Build history of the part. All positions in model axes, mm. A direction names the side the tool comes from. Give positions to 0.01 mm unless a question says otherwise; leave off trailing zeros. Order: outer loops, then holes, each group sorted by start corner. A loop starts at its lowest first (then second) coordinate and runs counter-clockwise, first axis right, second up. Notation, with made-up numbers: (45, -9) - (61, -9) arc R22 ccw to (61, 28) - close; hole circle Ø10 at (74.5, 22.5). An arc over 180 degrees is marked (long way). Use a Markdown table: item, result. Add a question column.
(1) Mould opens along Z. For faces 1 (the face through (59.49, 0.14, -11.07)), 2 (the face through (54.933, 0.14, -0.52)), 3 (the face through (0, 10, 53)) say: +Z half, -Z half, draft (parallel to the pull), parting line (faces both ways), or undercut.
(2) Flat gauge pins, fed straight in: pin 1 (4.5 mm diameter, centred on x = 57.28, z = 0, fed in from +Y); pin 2 (4 mm diameter, centred on x = 53, y = 2, fed in from +Z); pin 3 (5.5 mm diameter, centred on x = -57.28, z = 0, fed in from -Y); pin 4 (19.5 mm diameter, centred on x = -37.5, z = -36.5, fed in from -Y). Where does each tip first touch, or does it go through?
(3) Wall check: line 1 (X direction, y = 2.5, z = 0); line 2 (Y direction, x = -51.5, z = 16); line 3 (Z direction, x = 35.5, y = -1.5). Give the ranges that are in metal, low to high.
(4) Slice it at B-B (x = -26.5). Write the cut outline in (y, z).
(5) Slice it at D-D (y = -1). Write the cut outline in (x, z), then the cut area to 3 significant figures.
(6) Slice it at C-C (z = -15). Write the cut outline in (x, y), then the cut area to 3 significant figures.
(7) Slice it at A-A (z = 0). Write the cut outline in (x, y), then the cut area to 3 significant figures.
(8) Which spindle directions (+Z, -Z, +X, -X, +Y, -Y) get a long thin tool onto all of the face, cutting with end or side? Do faces 4 (the face through (55, -2, -12.5)), 5 (the face through (-55, -2, -12.5)), 6 (the face through (-55, -2, 12.5)), 7 (the face through (15, 3, -52)), 8 (the face through (55, -2, 12.5)). Say none if no direction does.
from build123d import *

# Parameters (mm, degrees)
BOSS_EXTRUDE1_DEPTH      = 10
BOSS_EXTRUDE1_DEPTH_BACK = 5
SKETCH1_R                = 55
SKETCH1_R_2              = 52.5
CUT_EXTRUDE2_DEPTH       = 80.214898
BOSS_EXTRUDE4_START      = -20
BOSS_EXTRUDE4_DEPTH      = 20
SKETCH7_R                = 2.4
CUT_EXTRUDE4_DEPTH       = 85.526942
FILLET1_R                = 5


with BuildPart() as part:
    # Sketch1 → Boss-Extrude1 (new, two sides: drawn at the far end of the back side and taken through both)
    with BuildSketch(Plane(origin=(0, 0, 0), x_dir=(1, 0, 0), z_dir=(0, 1, 0)).offset(-BOSS_EXTRUDE1_DEPTH_BACK)):
        with Locations(Location((0, 0, 0), (0, 0, 270))):
            Circle(SKETCH1_R)
        with Locations(Location((0, 0, 0), (0, 0, 270))):
            Circle(SKETCH1_R_2, mode=Mode.SUBTRACT)
    extrude(amount=BOSS_EXTRUDE1_DEPTH + BOSS_EXTRUDE1_DEPTH_BACK)

    # Sketch2 → Cut-Extrude2 (cut, through all)
    with BuildSketch(Plane(origin=(0, 10, 0), x_dir=(1, 0, 0), z_dir=(0, 1, 0))):
        Polygon((0, 0), (-15, 0), (-15, 70), (15, 70), (15, 0), align=None)
    extrude(amount=-CUT_EXTRUDE2_DEPTH, mode=Mode.SUBTRACT)

    # Sketch6 → Boss-Extrude4 (add)
    with BuildSketch(Plane(origin=(0, 10, 0), x_dir=(1, 0, 0), z_dir=(0, 1, 0)).offset(BOSS_EXTRUDE4_START)):
        with BuildLine():
            Line((50.990195, 12.5), (60.990195, 12.5))
            Line((60.990195, 12.5), (60.990195, -12.5))
            Line((60.990195, -12.5), (50.990195, -12.5))
            ThreePointArc((50.990195, -12.5), (52.5, 0), (50.990195, 12.5))
        make_face()
        with BuildLine():
            Line((-60.990195, -12.5), (-50.990195, -12.5))
            ThreePointArc((-50.990195, -12.5), (-52.5, 0), (-50.990195, 12.5))
            Line((-50.990195, 12.5), (-60.990195, 12.5))
            Line((-60.990195, 12.5), (-60.990195, -12.5))
        make_face()
    extrude(amount=BOSS_EXTRUDE4_DEPTH)

    # Sketch7 → Cut-Extrude4 (cut, through all)
    with BuildSketch(Plane(origin=(0, 10, 0), x_dir=(1, 0, 0), z_dir=(0, 1, 0))):
        with Locations(Location((-57.275454, 0, 0), (0, 0, 270))):
            Circle(SKETCH7_R)
        with Locations(Location((57.275454, 0, 0), (0, 0, 270))):
            Circle(SKETCH7_R)
    extrude(amount=-CUT_EXTRUDE4_DEPTH, mode=Mode.SUBTRACT)

    # Fillet1
    fillet1_edges = [part.edges().sort_by_distance(p)[0] for p in [
        (60.990195, 0, -12.5),
        (60.990195, 0, 12.5),
        (-60.990195, 0, 12.5),
        (-60.990195, 0, -12.5),
    ]]
    fillet(fillet1_edges, radius=FILLET1_R)


solid = part.part
Solution:
| question | item | result |
|---|---|---|
| 1 | face 1 | -Z half |
| 1 | face 2 | undercut |
| 1 | face 3 | draft |
| 2 | pin 1 | through |
| 2 | pin 2 | z = 20.59 |
| 2 | pin 3 | y = -10 |
| 2 | pin 4 | y = -5 |
| 3 | line 1 | -60.99 to -59.68, -54.88 to -52.5, 52.5 to 54.88, 59.68 to 60.99 |
| 3 | line 2 | -5 to 10 |
| 3 | line 3 | -42.01 to -38.68, 38.68 to 42.01 |
| 4 | outline | (-5, -48.19) - (10, -48.19) - (10, -45.32) - (-5, -45.32) - close; (-5, 45.32) - (10, 45.32) - (10, 48.19) - (-5, 48.19) - close |
| 5 | outline | (-60.99, -7.5) arc R5 ccw to (-55.99, -12.5) - (-53.56, -12.5) arc R55 ccw to (-15, -52.92) - (-15, -50.31) arc R52.5 cw (long way) to (15, -50.31) - (15, -52.92) arc R55 ccw to (53.56, -12.5) - (55.99, -12.5) arc R5 ccw to (60.99, -7.5) - (60.99, 7.5) arc R5 ccw to (55.99, 12.5) - (53.56, 12.5) arc R55 ccw to (-53.56, 12.5) - (-55.99, 12.5) arc R5 ccw to (-60.99, 7.5) - close; hole circle Ø4.8 at (-57.28, 0); hole circle Ø4.8 at (57.28, 0) |
| 5 | area | 1,030 mm2 |
| 6 | outline | (-52.92, -5) - (-50.31, -5) - (-50.31, 10) - (-52.92, 10) - close; (50.31, -5) - (52.92, -5) - (52.92, 10) - (50.31, 10) - close |
| 6 | area | 78.1 mm2 |
| 7 | outline | (-60.99, -10) - (-59.68, -10) - (-59.68, 10) - (-60.99, 10) - close; (-54.88, -10) - (-52.5, -10) - (-52.5, 10) - (-54.88, 10) - close; (52.5, -10) - (54.88, -10) - (54.88, 10) - (52.5, 10) - close; (59.68, -10) - (60.99, -10) - (60.99, 10) - (59.68, 10) - close |
| 7 | area | 148 mm2 |
| 8 | face 4 | -Z, +X, -Y |
| 8 | face 5 | -Z, -X, -Y |
| 8 | face 6 | +Z, -X, -Y |
| 8 | face 7 | -Z, +Y, -Y |
| 8 | face 8 | +Z, +X, -Y |
